Geometry check sheet. Reference: the model listing, model coordinates, mm. Face numbers are marked on the shaded views. Round coordinates to 2 decimals unless told otherwise and drop trailing zeros. Write each loop counter-clockwise with the first axis right and the second up, starting at its lowest first coordinate (ties: lowest second). Pieces come first, ordered by that corner, then holes. Notation, with made-up numbers: M -36,51.5 L -18,51.5 A25 cw -18,83.5 Z; hole C -24,-36 d5. An arc over 180 degrees is marked long. Put each result on its own line as item: value. Start each with the question number.
(1) Section check A-A on z = -9. Record the cut outline in (x, y).
(2) Gauge pin test, flat ends, axial feed: pin 1 (1.4 mm diameter, centred on x = -16.51, z = -25.4, fed in from +Y) (3 decimals); pin 2 (8 mm diameter, centred on x = 14.5, z = -4, fed in from -Y). Record the tip position at first contact, or that the pin passes through.
(3) Section check C-C on x = -5. Record the cut outline in (y, z), then the cut area to 3 significant figures.
(4) Material ranges on probe 1 along X at (y, z) = (-30, -16.5); probe 2 along Z at (x, y) = (8.5, -52); probe 3 along Z at (x, y) = (-17, -6), recorded low to high.
(5) Mould release check, pull along X, two halves, no side actions. Record for the marked faces 1, 2, 3 and 4: pulls with the +X half, pulls with the -X half, needs draft (parallel to the pull), parting line crosses it, or undercut.
from build123d import *

# Parameters (mm, degrees)
F1_DEPTH = 76.2
F2_R     = 1.26999


# Not quite as in the source:
# - a fillet or chamfer is up to 0.001 mm smaller than in the source, because OpenCascade refuses the exact size


with BuildPart() as f1:
    # F0 (on Front) → F1 (new body)
    with BuildSketch(Plane.XZ):
        with BuildLine():
            Line((-16.51, 19.05), (-19.05, 19.05))
            Line((-19.05, 19.05), (-19.05, -30.1625))
            Line((-19.05, -30.1625), (0, -30.1625))
            Line((0, -30.1625), (0, -25.4))
            Line((0, -25.4), (-15.71625, -25.4))
            ThreePointArc((-15.71625, -25.4), (-17.0712660076, -25.9612660076), (-16.51, -24.60625))
            Line((-16.51, -24.60625), (-16.51, 19.05))
        make_face()
        with BuildLine():
            Line((0, -25.4), (0, -30.1625))
            Line((0, -30.1625), (19.05, -30.1625))
            Line((19.05, -30.1625), (19.05, 19.05))
            Line((19.05, 19.05), (16.51, 19.05))
            Line((16.51, 19.05), (16.51, -24.60625))
            ThreePointArc((16.51, -24.60625), (17.0712660076, -24.8387339924), (17.30375, -25.4))
            ThreePointArc((17.30375, -25.4), (16.51, -26.19375), (15.71625, -25.4))
            Line((15.71625, -25.4), (0, -25.4))
        make_face()
    extrude(amount=F1_DEPTH)

    # F2 (radius 1.27 in the source; OpenCascade refuses exactly that, so slightly less here)
    f2_edges = [f1.edges().sort_by_distance(p)[0] for p in [
        (19.05, -38.1, 19.05),
        (16.51, -38.1, 19.05),
        (17.78, 0, 19.05),
        (17.78, -76.2, 19.05),
        (-16.51, -38.1, 19.05),
        (-19.05, -38.1, 19.05),
        (-17.78, 0, 19.05),
        (-17.78, -76.2, 19.05),
        (-19.05, -76.2, -5.55625),
        (19.05, -76.2, -5.55625),
        (19.05, 0, -5.55625),
        (-19.05, 0, -5.55625),
        (-19.05, -38.1, -30.1625),
        (19.05, -38.1, -30.1625),
        (0, 0, -30.1625),
        (0, -76.2, -30.1625),
    ]]
    fillet(f2_edges, radius=F2_R)


solid = f1.part
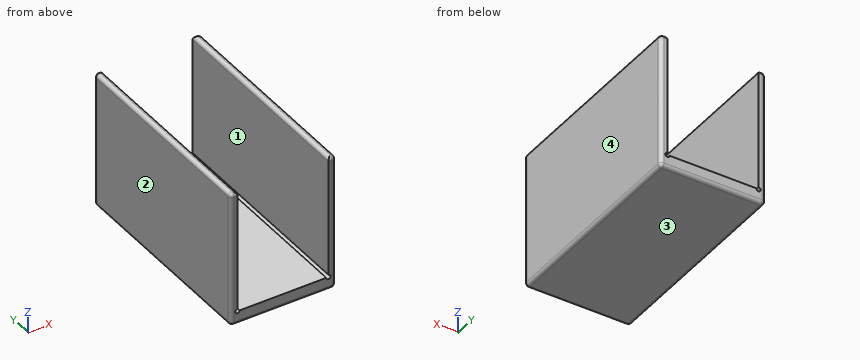
Answers follow:
1. outline: M -19.05,-74.93 A1.27 ccw -17.78,-76.2 L -16.51,-76.2 L -16.51,0 L -17.78,0 A1.27 ccw -19.05,-1.27 Z; M 16.51,-76.2 L 17.78,-76.2 A1.27 ccw 19.05,-74.93 L 19.05,-1.27 A1.27 ccw 17.78,0 L 16.51,0 Z
2. pin 1: passes through
2. pin 2: stops at y = -76.2
3. outline: M -76.2,-28.89 A1.27 ccw -74.93,-30.16 L -1.27,-30.16 A1.27 ccw 0,-28.89 L 0,-25.4 L -76.2,-25.4 Z
3. area: 362 mm^2
4. probe 1: x = -19.05 to -16.51, 16.51 to 19.05
4. probe 2: z = -30.16 to -25.4
4. probe 3: z = -30.16 to -26.02, -24.78 to 18.78
5. face 1: undercut
5. face 2: pulls with the -X half
5. face 3: needs draft
5. face 4: pulls with the +X half
